For this review, take the finished solid that the model builds, in its own axes (mm). A direction names the side the tool comes from. Coordinates: 2 decimals unless noted, no trailing zeros. Write each loop counter-clockwise with the first axis right and the second up, starting at its lowest first coordinate (ties: lowest second). Pieces come first, ordered by that corner, then holes.
1) We need section C-C on z = -7.5. Write out the cut boundary in (x, y).
2) We need section D-D on y = 5.75. Write out the cut boundary in (x, z), then the cut area to 3 significant figures.
3) Insertion check: P1, Ø1.5, axis at y = -2, z = -4.5, coming from the -X side; P2, Ø10, axis at x = -3.5, z = -5.5, coming from the +Y side; P3, Ø4, axis at x = -1.5, z = -8, coming from the -Y side. Each pin has a flat end and moves straight along its axis. Give the tip position at first contact, or say it passes through.
4) To check wall thickness, follow line 1 along X through (y, z) = (1.5, -5.75); line 2 along Y through (x, z) = (-5.75, -10.25); line 3 along Z through (x, y) = (9, 5.5). State the ranges of each line that lie inside material, in increasing order.
5) We need section B-B on x = -0.75. Write out the cut boundary in (y, z).
6) We need section A-A on y = 1.75. Write out the cut boundary in (x, z), then the cut area to 3 significant figures.
7) For faces 1 (the face through (0, -5.08, -6)), 2 (the face through (-11.43, 0, -6)), 3 (the face through (0, 5.08, -6)), list the 3-axis set-ups (+Z, -Z, +X, -X, +Y, -Y) from which the entire face can be reached by the end or side of a thin tool; tool diameter is ignored.
from build123d import *

# Parameters (mm, degrees)
SKETCH1_W           = 22.86
SKETCH1_H           = 10.16
BOSS_EXTRUDE1_DEPTH = 12.7
SKETCH2_W           = 25.4
SKETCH2_H           = 12.7
BOSS_EXTRUDE2_DEPTH = 6.35


with BuildPart() as part:
    # Sketch1 → Boss-Extrude1 (new body)
    with BuildSketch(Plane.XY):
        Rectangle(SKETCH1_W, SKETCH1_H)
    extrude(amount=-BOSS_EXTRUDE1_DEPTH)

    # Sketch2 → Boss-Extrude2 (add)
    with BuildSketch(Plane.XY):
        Rectangle(SKETCH2_W, SKETCH2_H)
    extrude(amount=BOSS_EXTRUDE2_DEPTH)


solid = part.part
Result:
1. outline: (-11.43, -5.08) - (11.43, -5.08) - (11.43, 5.08) - (-11.43, 5.08) - close
2. outline: (-12.7, 0) - (12.7, 0) - (12.7, 6.35) - (-12.7, 6.35) - close
2. area: 161 mm2
3. P1: stops at x = -11.43
3. P2: stops at y = 5.08
3. P3: stops at y = -5.08
4. line 1: x = -11.43 to 11.43
4. line 2: y = -5.08 to 5.08
4. line 3: z = 0 to 6.35
5. outline: (-6.35, 0) - (-5.08, 0) - (-5.08, -12.7) - (5.08, -12.7) - (5.08, 0) - (6.35, 0) - (6.35, 6.35) - (-6.35, 6.35) - close
6. outline: (-12.7, 0) - (-11.43, 0) - (-11.43, -12.7) - (11.43, -12.7) - (11.43, 0) - (12.7, 0) - (12.7, 6.35) - (-12.7, 6.35) - close
6. area: 452 mm2
7. face 1: -Z, +X, -X, -Y
7. face 2: -Z, -X, +Y, -Y
7. face 3: -Z, +X, -X, +Y
